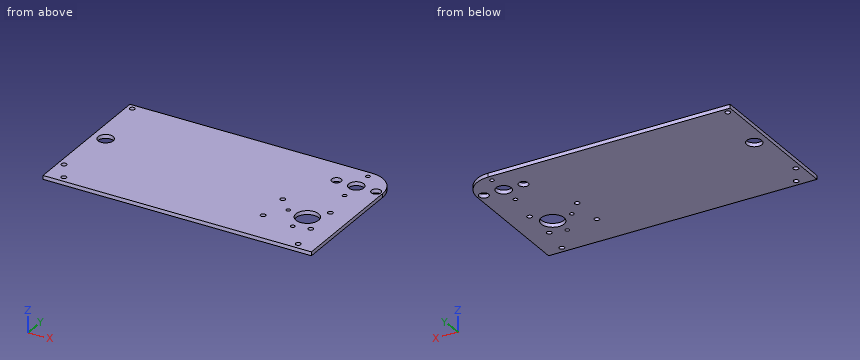
from build123d import *

# Parameters (mm, degrees)
F0_R     = 2.15265
F0_R_2   = 2.1
F0_R_3   = 1.7272
F0_R_4   = 9.587497
F0_R_5   = 6.35
F0_R_6   = 3.96875
F1_DEPTH = 3.175


with BuildPart() as f1:
    # F0 (on Top) → F1 (new body)
    with BuildSketch(Plane.XY):
        with BuildLine():
            Line((0, 22.225), (-203.2, 22.225))
            Line((-203.2, 22.225), (-203.2, -101.6))
            Line((-203.2, -101.6), (22.225, -101.6))
            Line((22.225, -101.6), (22.225, -90.805))
            Line((22.225, -90.805), (22.225, 0))
            ThreePointArc((22.225, 0), (15.715448, 15.715448), (0, 22.225))
        make_face()
        with Locations((-188.9125, -96.2025)):
            Circle(F0_R, mode=Mode.SUBTRACT)
        with Locations((-198.4375, -79.6925)):
            Circle(F0_R, mode=Mode.SUBTRACT)
        with Locations((-35.729847, -72.110361)):
            Circle(F0_R_2, mode=Mode.SUBTRACT)
        with Locations((7.9375, -96.2025)):
            Circle(F0_R, mode=Mode.SUBTRACT)
        with Locations((-8.920831, -75.349563)):
            Circle(F0_R_3, mode=Mode.SUBTRACT)
        with Locations((4.270153, -72.110361)):
            Circle(F0_R_2, mode=Mode.SUBTRACT)
        with Locations((-35.729847, -44.110361)):
            Circle(F0_R_2, mode=Mode.SUBTRACT)
        with Locations((-24.119039, -56.069367)):
            Circle(F0_R_3, mode=Mode.SUBTRACT)
        with Locations((-6.879837, -58.110361)):
            Circle(F0_R_4, mode=Mode.SUBTRACT)
        with Locations((4.270153, -44.110361)):
            Circle(F0_R_2, mode=Mode.SUBTRACT)
        with Locations((-192.0875, -31.115)):
            Circle(F0_R_5, mode=Mode.SUBTRACT)
        with Locations((-198.4375, 17.4625)):
            Circle(F0_R, mode=Mode.SUBTRACT)
        with Locations((0, -16.66875)):
            Circle(F0_R_3, mode=Mode.SUBTRACT)
        with Locations((-16.66875, 0)):
            Circle(F0_R_6, mode=Mode.SUBTRACT)
        Circle(F0_R_5, mode=Mode.SUBTRACT)
        with Locations((16.66875, 0)):
            Circle(F0_R_6, mode=Mode.SUBTRACT)
        with Locations((0, 16.66875)):
            Circle(F0_R_3, mode=Mode.SUBTRACT)
    extrude(amount=F1_DEPTH)


solid = f1.part
Design review of the part built by this model. Coordinates are the model's own, in mm. Coordinates: 2 decimals unless noted, no trailing zeros. Use one line per item in the form item = value. Start each with the question number.
(1) Add section A-A on z = 0.6. Give the number of separate pieces and of enclosed holes in the cut face, plus the area to 3 significant figures.
(2) Insertion check: pin 1 (3 mm diameter, centred on x = -8.92, y = -75.35, fed in from +Z). The pin has a flat end and moves straight along its axis. Give the tip position at first contact, or say it passes through.
(3) For probe 1 along X at (y, z) = (-96, 1.8) (3 decimals); probe 2 along X at (y, z) = (-58.5, 1.1) (3 decimals); probe 3 along Y at (x, z) = (-16.5, 2.35) (3 decimals), list the stretches that pass through material, from the lowest coordinate up.
Answer block:
q1.separate_pieces = 1
q1.enclosed_holes = 17
q1.area = 27,000 mm²
q2.pin_1 = through
q3.probe_1 = -203.2 to -191.056, -186.769 to 5.794, 10.081 to 22.225
q3.probe_2 = -203.2 to -16.459, 2.7 to 22.225
q3.probe_3 = -101.6 to -3.965, 3.965 to 22.225
